```python
from build123d import *

# Parameters (mm, degrees)
SKETCH1_W               = 17
SKETCH1_H               = 15
BOSS_EXTRUDE1_DEPTH     = 5
SKETCH2_W               = 3
SKETCH2_H               = 15
SKETCH2_H_2             = 14.97636143
BOSS_EXTRUDE2_DEPTH     = 5
CUT_EXTRUDE2_DEPTH      = 21.185301583
CUT_EXTRUDE2_DEPTH_BACK = 21.185301583
SKETCH4_R               = 1.5
FILLET1_R               = 6
FILLET3_RADIUS          = 1.5
FILLET3_LENGTH          = 14.97636143
FILLET4_RADIUS          = 1.5
FILLET4_LENGTH          = 15


with BuildPart() as part:
    # Sketch1 → Boss-Extrude1 (new body)
    with BuildSketch(Plane.XY):
        with Locations((-8.5, -7.5)):
            Rectangle(SKETCH1_W, SKETCH1_H)
    extrude(amount=BOSS_EXTRUDE1_DEPTH)

    # Sketch2 → Boss-Extrude2 (add)
    with BuildSketch(Plane.XY.offset(5)):
        with Locations((-6.42, -7.5)):
            Rectangle(SKETCH2_W, SKETCH2_H)
        with Locations((-10.58, -7.511819285)):
            Rectangle(SKETCH2_W, SKETCH2_H_2)
    extrude(amount=BOSS_EXTRUDE2_DEPTH)

    # Sketch4 → Cut-Extrude2 (cut, two sides: drawn at the far end of the back side and taken through both)
    with BuildSketch(Plane(origin=(-9.08, 0, 0), x_dir=(0, 0, -1), z_dir=(1, 0, 0)).offset(-CUT_EXTRUDE2_DEPTH_BACK)):
        with Locations(Location((-7.041389116, -7.762480296, 0), (0, 0, 270))):
            Circle(SKETCH4_R)
    extrude(amount=CUT_EXTRUDE2_DEPTH + CUT_EXTRUDE2_DEPTH_BACK, mode=Mode.SUBTRACT)

    # Fillet1
    # the kernel refuses this fillet: 6 mm, written as the material it takes off along each edge
    with BuildSketch(Plane(origin=(0, -29.754999153, 5), x_dir=(0, 0, -1), z_dir=(0, 1, 0))) as fillet1_piece_1:
        with BuildLine():
            CenterArc((5.901999661, 6), FILLET1_R, 190.369759805, 79.630240195)
            Line((0, 4.92), (0, 0))
            Line((0, 0), (5.901999661, 0))
        make_face()
    extrude(amount=44.509998306, mode=Mode.SUBTRACT)
    # the kernel refuses this fillet: 6 mm, written as the material it takes off along each edge
    with BuildSketch(Plane(origin=(-17, 14.790199458, 5), x_dir=(0, 0, -1), z_dir=(0, -1, 0))) as fillet1_2_piece_1_section:
        with BuildLine():
            CenterArc((6, 5.916079783), FILLET1_R, 180, 80.405931773)
            Line((0, 5.916079783), (0, 0))
            Line((0, 0), (5, 0))
        make_face()
    fillet1_2_piece_1 = extrude(amount=44.580398916, mode=Mode.PRIVATE)
    fillet1_2_piece_1 = split(fillet1_2_piece_1, bisect_by=Plane(origin=(-17, -0.02363857, 5), z_dir=(0, 1, 0)), keep=Keep.TOP, mode=Mode.PRIVATE)
    fillet1_2_piece_1 = split(fillet1_2_piece_1, bisect_by=Plane(origin=(-12.08, 14.790199458, 5), z_dir=(-1, 0, 0)), keep=Keep.TOP, mode=Mode.PRIVATE)
    add(fillet1_2_piece_1, mode=Mode.SUBTRACT)
    with BuildSketch(Plane(origin=(-17, 14.790199458, 5), x_dir=(0, 0, -1), z_dir=(0, -1, 0))) as fillet1_2_piece_2_section:
        with BuildLine():
            CenterArc((6, 5.916079783), FILLET1_R, 180, 80.405931773)
            Line((0, 5.916079783), (0, 0))
            Line((0, 0), (5, 0))
        make_face()
    fillet1_2_piece_2 = extrude(amount=44.580398916, mode=Mode.PRIVATE)
    fillet1_2_piece_2 = split(fillet1_2_piece_2, bisect_by=Plane(origin=(-17, -0.02363857, 5), z_dir=(0, 1, 0)), keep=Keep.TOP, mode=Mode.PRIVATE)
    fillet1_2_piece_2 = split(fillet1_2_piece_2, bisect_by=Plane(origin=(-12.08, 14.790199458, 5), z_dir=(1, 0, 0)), keep=Keep.TOP, mode=Mode.PRIVATE)
    add(fillet1_2_piece_2, mode=Mode.SUBTRACT)
    with BuildSketch(Plane(origin=(-17, 14.790199458, 5), x_dir=(0, 0, -1), z_dir=(0, -1, 0))) as fillet1_2_piece_3_section:
        with BuildLine():
            CenterArc((6, 5.916079783), FILLET1_R, 180, 80.405931773)
            Line((0, 5.916079783), (0, 0))
            Line((0, 0), (5, 0))
        make_face()
    fillet1_2_piece_3 = extrude(amount=44.580398916, mode=Mode.PRIVATE)
    fillet1_2_piece_3 = split(fillet1_2_piece_3, bisect_by=Plane(origin=(-17, -0.02363857, 5), z_dir=(0, -1, 0)), keep=Keep.TOP, mode=Mode.PRIVATE)
    fillet1_2_piece_3 = split(fillet1_2_piece_3, bisect_by=Plane(origin=(-12.08, 14.790199458, 5), z_dir=(-1, 0, 0)), keep=Keep.TOP, mode=Mode.PRIVATE)
    add(fillet1_2_piece_3, mode=Mode.SUBTRACT)

    # Fillet3: full round fillet: the end face becomes a half cylinder, R = half its width
    fillet3_face = Plane((-10.58, -7.511819285, 10), x_dir=(0, -1, 0), z_dir=(0, 0, 1))  # on the end face: x along it, z out of the body
    fillet3_slab = fillet3_face.offset(-FILLET3_RADIUS / 2) * Box(FILLET3_LENGTH, 2 * FILLET3_RADIUS, FILLET3_RADIUS, mode=Mode.PRIVATE)  # the body's end, R deep
    fillet3_round = Plane((-10.58, -7.511819285, 8.5), x_dir=(0, 0, 1), z_dir=(0, -1, 0)) * Cylinder(FILLET3_RADIUS, FILLET3_LENGTH, mode=Mode.PRIVATE)  # its axis R under the face
    add(fillet3_slab - fillet3_round, mode=Mode.SUBTRACT)

    # Fillet4: full round fillet: the end face becomes a half cylinder, R = half its width
    fillet4_face = Plane((-6.42, -7.5, 10), x_dir=(0, -1, 0), z_dir=(0, 0, 1))  # on the end face: x along it, z out of the body
    fillet4_slab = fillet4_face.offset(-FILLET4_RADIUS / 2) * Box(FILLET4_LENGTH, 2 * FILLET4_RADIUS, FILLET4_RADIUS, mode=Mode.PRIVATE)  # the body's end, R deep
    fillet4_round = Plane((-6.42, -7.5, 8.5), x_dir=(0, 0, 1), z_dir=(0, -1, 0)) * Cylinder(FILLET4_RADIUS, FILLET4_LENGTH, mode=Mode.PRIVATE)  # its axis R under the face
    add(fillet4_slab - fillet4_round, mode=Mode.SUBTRACT)


solid = part.part
```
The model under review builds one solid part; all positions refer to its coordinate system, in mm. A direction names the side the tool comes from. Round coordinates to 2 decimals unless told otherwise and drop trailing zeros. Loops run counter-clockwise (first coordinate to the right, second up) from the corner with the lowest first, then second, coordinate; pieces in that order, holes last. Notation, with made-up numbers: (51.5, 17) -> (91.5, 17) arc R15 cw to (91.5, 25) -> close; hole circle Ø11 at (25.25, 41). An arc over 180 degrees is marked (long way). Answer in a Markdown table with one row per item.
1) Draft analysis for pull direction X (two halves, no side actions). For faces 6 (the cylindrical face through (-14.91, -7.4, 3.62)), 7 (the flat face through (-7.92, -7.6, 5.2)), 8 (the flat face through (-11, -0.024, 7)), state which applies: pulls with the +X half, pulls with the -X half, needs draft (parallel to the pull), parting line crosses it, or undercut.
Taken from the geometry:
| item | result |
|---|---|
| face 6 | pulls with the -X half |
| face 7 | undercut |
| face 8 | needs draft |
2) For pin 1 Ø3.5 at (y, z) = (-7.76, 7.04) entering from +X; pin 2 Ø3.5 at (x, z) = (-10.5, 8) entering from +Y; pin 3 Ø6 at (y, z) = (-6, 1.5) entering from -X, all flat-tipped, find the tip position at first contact; note any pin that passes through.
Taken from the geometry:
| item | result |
|---|---|
| pin 1 | stops at x = -4.92 |
| pin 2 | stops at y = -0.02 |
| pin 3 | stops at x = -17 |
3) Consider section D-D, the plane y = -10. Write out the cut boundary in (x, z).
Taken from the geometry:
| item | result |
|---|---|
| outline | (-17, 0) -> (-0.07, 0) arc R6 ccw to (-4.92, 5) -> (-4.92, 8.5) arc R1.5 ccw to (-7.92, 8.5) -> (-7.92, 5) -> (-9.08, 5) -> (-9.08, 8.5) arc R1.5 ccw to (-12.08, 8.5) -> (-12.08, 4.92) arc R6 ccw to start |
4) Wall thickness on line 1 along X through (y, z) = (-2.25, 7); line 2 along Y through (x, z) = (-11.5, 7.5); line 3 along Z through (x, y) = (-10.5, -9.75): over which ranges is each line inside the solid? List them lowest first.
Taken from the geometry:
| item | result |
|---|---|
| line 1 | x = -12.08 to -9.08, -7.92 to -4.92 |
| line 2 | y = -15 to -9.19, -6.33 to -0.02 |
| line 3 | z = 0 to 10 |
5) Consider section B-B, the plane z = 8.75. Write out the cut boundary in (x, y), plus the area to 3 significant figures.
Taken from the geometry:
| item | result |
|---|---|
| outline | (-12.06, -15) -> (-9.1, -15) -> (-9.1, -0.02) -> (-12.06, -0.02) -> close; (-7.9, -15) -> (-4.94, -15) -> (-4.94, 0) -> (-7.9, 0) -> close |
| area | 88.7 mm² |
6) Consider section A-A, the plane y = -7.75. Write out the cut boundary in (x, z).
Taken from the geometry:
| item | result |
|---|---|
| outline | (-17, 0) -> (-0.07, 0) arc R6 ccw to (-4.92, 5) -> (-4.92, 5.54) -> (-7.92, 5.54) -> (-7.92, 5) -> (-9.08, 5) -> (-9.08, 5.54) -> (-12.08, 5.54) -> (-12.08, 4.92) arc R6 ccw to start; (-12.08, 8.54) -> (-9.08, 8.54) arc R1.5 ccw to start; (-7.92, 8.54) -> (-4.92, 8.54) arc R1.5 ccw to start |
7) Tool access review of faces 1 (the flat face through (-9, -15, 4)), 2 (the flat face through (-9.08, -7.6, 5.2)), 3 (the flat face through (-12.08, -7.6, 5.1)), 4 (the flat face through (-4.92, -7.6, 5.2)), 5 (the flat face through (-9, -7, 0)): name each direction out of +Z, -Z, +X, -X, +Y, -Y from which nothing blocks a thin tool from reaching the whole face with its end or side.
Taken from the geometry:
| item | result |
|---|---|
| face 1 | +Z, -Z, +X, -X, -Y |
| face 2 | +Z, +Y, -Y |
| face 3 | +Z, -X, +Y, -Y |
| face 4 | +Z, +X, +Y, -Y |
| face 5 | -Z, +X, -X, +Y, -Y |
